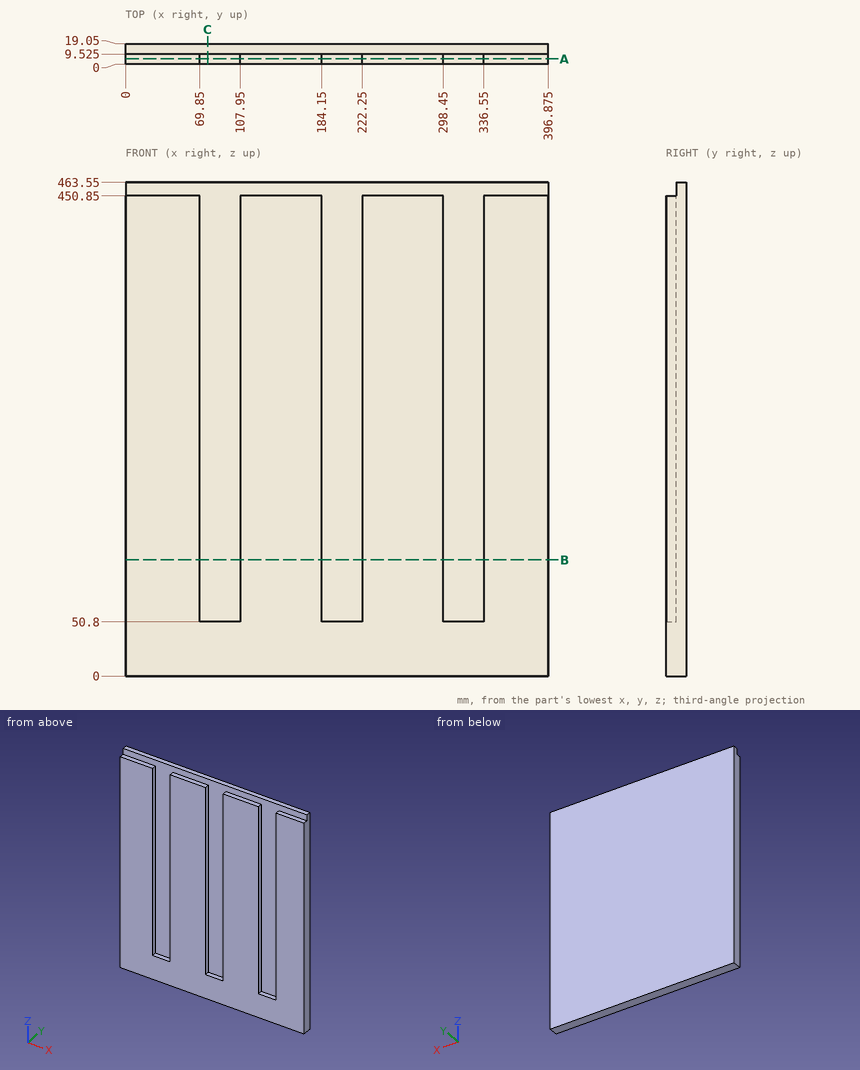
Study the drawing (mm; zero at the part's minimum x, y, z) and answer. Coordinates: 2 decimals unless noted, no trailing zeros. Loops run counter-clockwise (first coordinate to the right, second up) from the corner with the lowest first, then second, coordinate; pieces in that order, holes last. Notation, with made-up numbers: (-29, 31) -> (-9, 31) arc R28 ccw to (-9, 51) -> close; hole circle Ø1 at (58.25, 66.5). An arc over 180 degrees is marked (long way). Write each question's results on one line, items separated by ' | '. Start each with the question number.
1) Find section A-A on y = 5. Determine the outline of the cut face in (x, z) (3 decimals), then the cut area to 3 significant figures.
2) Find section C-C on x = 77. Determine the outline of the cut face in (y, z) (3 decimals).
3) Flat-ended cylindrical pins translate along their axes: P1, Ø7.5, axis at x = 378, y = 7, coming from the +Z side; P2, Ø5, axis at x = 89, y = 3, coming from the +Z side; P3, Ø3, axis at x = 48.5, y = 4, coming from the +Z side. Find the tip coordinate at first contact, or state that the pin passes through.
4) Consider line 1 along X through (y, z) = (5.5, 374) (3 decimals); line 2 along Z through (x, y) = (67.5, 5.5); line 3 along Z through (x, y) = (322.5, 3.75). Determine where each line is inside the solid, lowest interval first.
5) Find section B-B on z = 109. Determine the outline of the cut face in (x, y) (3 decimals).
Response values:
1) outline: (0, 0) -> (396.875, 0) -> (396.875, 450.85) -> (336.55, 450.85) -> (336.55, 50.8) -> (298.45, 50.8) -> (298.45, 450.85) -> (222.25, 450.85) -> (222.25, 50.8) -> (184.15, 50.8) -> (184.15, 450.85) -> (107.95, 450.85) -> (107.95, 50.8) -> (69.85, 50.8) -> (69.85, 450.85) -> (0, 450.85) -> close | area: 133,000 mm^2
2) outline: (0, 0) -> (19.05, 0) -> (19.05, 463.55) -> (9.525, 463.55) -> (9.525, 50.8) -> (0, 50.8) -> close
3) P1: stops at z = 463.55 | P2: stops at z = 50.8 | P3: stops at z = 450.85
4) line 1: x = 0 to 69.85, 107.95 to 184.15, 222.25 to 298.45, 336.55 to 396.875 | line 2: z = 0 to 450.85 | line 3: z = 0 to 50.8
5) outline: (0, 0) -> (69.85, 0) -> (69.85, 9.525) -> (107.95, 9.525) -> (107.95, 0) -> (184.15, 0) -> (184.15, 9.525) -> (222.25, 9.525) -> (222.25, 0) -> (298.45, 0) -> (298.45, 9.525) -> (336.55, 9.525) -> (336.55, 0) -> (396.875, 0) -> (396.875, 19.05) -> (0, 19.05) -> close
